```python
from build123d import *

# Parameters (mm, degrees)
BOSS_EXTRUDE1_DEPTH = 4
SKETCH10_R          = 1.5
SKETCH10_W          = 40
SKETCH10_H          = 6.922711204
CUT_EXTRUDE2_DEPTH  = 31.436460939


with BuildPart() as part:
    # Sketch1 → Boss-Extrude1 (new, symmetric)
    with BuildSketch(Plane(origin=(0, 0, 0), x_dir=(1, 0, 0), z_dir=(0, 1, 0))):
        with BuildLine():
            Line((-20, 0), (0, 0))
            Line((0, 0), (20, 0))
            Line((20, 0), (20, -8))
            Line((20, -8), (24, -8))
            Line((24, -8), (24, -16.922711204))
            ThreePointArc((24, -16.922711204), (0, -14), (-24, -16.922711204))
            Line((-24, -16.922711204), (-24, -8))
            Line((-24, -8), (-20, -8))
            Line((-20, -8), (-20, 0))
        make_face()
    extrude(amount=BOSS_EXTRUDE1_DEPTH, both=True)

    # Sketch10 → Cut-Extrude2 (cut, through all)
    with BuildSketch(Plane(origin=(0, 4, 0), x_dir=(1, 0, 0), z_dir=(0, 1, 0))):
        with Locations(Location((-12.5, -9.922711204, 0), (0, 0, 270))):
            Circle(SKETCH10_R)
        with Locations(Location((12.5, -9.922711204, 0), (0, 0, 270))):
            Circle(SKETCH10_R)
        with Locations((0, -3.461355602)):
            Rectangle(SKETCH10_W, SKETCH10_H)
    extrude(amount=-CUT_EXTRUDE2_DEPTH, mode=Mode.SUBTRACT)


solid = part.part
```
Model file for the job. Use its own axes, mm. A direction names the side the tool comes from. Round coordinates to 2 decimals unless told otherwise and drop trailing zeros. Order: outer loops, then holes, each group sorted by start corner. A loop starts at its lowest first (then second) coordinate and runs counter-clockwise, first axis right, second up. Notation, with made-up numbers: (-25, 40) -> (1, 40) arc R11 cw to (1, 49) -> close; hole circle Ø3 at (66, 9). An arc over 180 degrees is marked (long way). Use one line per item in the form item = value.
Item 1: Drill centre lines: line 1 (X direction, y = 3.25, z = 10); line 2 (X direction, y = 3.75, z = 10.5); line 3 (Z direction, x = 1, y = 0.25) (3 decimals). Where is each one in solid material? Low to high.
Returned:
line_1 = -24 to -14, -11 to 11, 14 to 24
line_2 = -24 to -13.88, -11.12 to 11.12, 13.88 to 24
line_3 = 6.923 to 14.005
Item 2: Cut at B-B, the plane x = 13. Write the cut outline in (y, z).
Returned:
outline = (-4, 6.92) -> (4, 6.92) -> (4, 8.51) -> (-4, 8.51) -> close; (-4, 11.34) -> (4, 11.34) -> (4, 14.85) -> (-4, 14.85) -> close
Item 3: Tool access for faces 1 (the face through (0, 4, 11)), 2 (the face through (-20, 0.1, 7.5)), 3 (the face through (20, 0.1, 7.5)): list every direction of +Z, -Z, +X, -X, +Y, -Y with a clear straight run to the whole face (end or side of a thin tool).
Returned:
face_1 = +Z, -Z, +X, -X, +Y
face_2 = -Z, -X, +Y, -Y
face_3 = -Z, +X, +Y, -Y
Item 4: Flat gauge pins, fed straight in: pin 1 Ø2.5 at (x, z) = (12.5, 9.92) entering from -Y; pin 2 Ø1.2 at (x, y) = (-21.5, -1) entering from -Z. Where does each tip first touch, or does it go through?
Returned:
pin_1 = through
pin_2 = 8
Item 5: Cut at A-A, the plane y = 2. Write the cut outline in (x, z), and give its area (3 significant figures).
Returned:
outline = (-24, 8) -> (-20, 8) -> (-20, 6.92) -> (20, 6.92) -> (20, 8) -> (24, 8) -> (24, 16.92) arc R100 cw to (-24, 16.92) -> close; hole circle Ø3 at (-12.5, 9.92); hole circle Ø3 at (12.5, 9.92)
area = 363 mm^2
Item 6: Cut at C-C, the plane z = 9. Write the cut outline in (x, y).
Returned:
outline = (-24, -4) -> (-13.68, -4) -> (-13.68, 4) -> (-24, 4) -> close; (-11.32, -4) -> (11.32, -4) -> (11.32, 4) -> (-11.32, 4) -> close; (13.68, -4) -> (24, -4) -> (24, 4) -> (13.68, 4) -> close
Item 7: Pull direction Z, two halves, no side cores. Call faces 4 (the face through (-13.07, 0.06, 11.31)), 5 (the face through (11.93, 0.06, 11.31)), 6 (the face through (0, 0, 14)), 7 (the face through (22, 0, 8)): released by +Z, released by -Z, zero draft, split by the parting line, or undercut.
Returned:
face_4 = undercut
face_5 = undercut
face_6 = released by +Z
face_7 = released by -Z
Item 8: Cut at D-D, the plane x = -12. Write the cut outline in (y, z), and give its area (3 significant figures).
Returned:
outline = (-4, 6.92) -> (4, 6.92) -> (4, 8.51) -> (-4, 8.51) -> close; (-4, 11.34) -> (4, 11.34) -> (4, 14.72) -> (-4, 14.72) -> close
area = 39.8 mm^2
